Autodesk Inventor part; units mm, degrees
ref_plane "YZ Plane" through (0, 0, 0) normal (1, 0, 0) x (0, 1, 0)
ref_plane "XZ Plane" through (0, 0, 0) normal (0, 1, 0) x (-1, 0, 0)
ref_plane "XY Plane" through (0, 0, 0) normal (0, 0, 1) x (1, 0, 0)
sketch "Sketch1" plane through (0, 0, 0) normal (0, 1, 0) x (-1, 0, 0)
  line L0 (-152.4, -228.6) -> (152.4, -228.6)
  line L1 (152.4, -228.6) -> (152.4, 228.6)
  line L2 (152.4, 228.6) -> (-152.4, 228.6)
  line L3 (-152.4, 228.6) -> (-152.4, -228.6)
  line L4 (-152.4, -228.6) -> (152.4, 228.6) construction
  line L5 (152.4, -228.6) -> (-152.4, 228.6) construction
  point P0 (0, 0)
  dimension "d0" = 457.2
  dimension "d1" = 304.8
extrude "Extrusion1" add sketch "Sketch1" against normal blind 19.05
sketch "Sketch3" plane through (0, -19.05, 0) normal (0, -1, 0) x (1, 0, 0)
  line L0 (152.4, -228.6) -> (152.4, 228.6)
  line L1 (-152.4, 228.6) -> (-152.4, -228.6)
  line L2 (152.4, 228.6) -> (-152.4, 228.6)
  line L3 (-152.4, 228.6) -> (-152.4, 190.5)
  line L4 (-152.4, 190.5) -> (152.4, 190.5)
  line L5 (152.4, 190.5) -> (152.4, 228.6)
  line L6 (-152.4, -228.6) -> (152.4, -228.6)
  line L7 (152.4, -190.5) -> (-152.4, -190.5)
  line L8 (-152.4, -190.5) -> (-152.4, -228.6)
  line L9 (-152.4, -228.6) -> (152.4, -228.6)
  line L10 (152.4, -228.6) -> (152.4, -190.5)
  point P0 (0, 0)
  dimension "d4" = 38.1
  dimension "d5" = 38.1
extrude "Extrusion2" add sketch "Sketch3" along normal blind 38.1 contours L6 L1 L7 L0 | L4 L1 L2 L0
sketch "Sketch4" plane through (0, 0, 0) normal (0, 1, 0) x (1, 0, 0)
  line L0 (-152.4, -228.6) -> (152.4, -228.6)
  line L1 (-72.2315, -228.6) -> (72.2315, -228.6)
  line L2 (72.2315, -228.6) -> (72.2315, 76.2)
  line L3 (72.2315, 76.2) -> (-72.2315, 76.2)
  line L4 (-72.2315, 76.2) -> (-72.2315, -228.6)
  line L5 (-152.4, 228.6) -> (-152.4, -228.6)
  point P0 (0, 0)
  dimension "d8" = 144.463
  dimension "d9" = 304.8
  dimension "d10" = 80.1685
extrude "Extrusion3" cut sketch "Sketch4" against normal blind 19.05
sketch "Sketch5" plane through (0, 0, 0) normal (0, 1, 0) x (1, 0, 0)
  line L0 (-102.4, 228.6) -> (-65.887, 228.6)
  line L1 (-65.887, 228.6) -> (-65.887, 206.6)
  line L2 (-65.887, 206.6) -> (-102.4, 206.6)
  line L3 (-102.4, 206.6) -> (-102.4, 228.6)
  line L4 (152.4, 228.6) -> (-152.4, 228.6)
  line L5 (65.887, 228.6) -> (102.4, 228.6)
  line L6 (102.4, 228.6) -> (102.4, 206.6)
  line L7 (102.4, 206.6) -> (65.887, 206.6)
  line L8 (65.887, 206.6) -> (65.887, 228.6)
  line L9 (-152.4, 228.6) -> (-152.4, -228.6)
  line L10 (152.4, -228.6) -> (152.4, 228.6)
  point P0 (0, 0)
  point P1 (-65.887, 217.6)
  point P2 (84.1435, 228.6)
  dimension "d13" = 0
  dimension "d14" = 36.513
  dimension "d15" = 22
  dimension "d16" = 36.513
  dimension "d17" = 22
  dimension "d18" = 50
  dimension "d19" = 50
extrude "Extrusion4" cut sketch "Sketch5" against normal blind 5
properties material "Wood (Maple)"
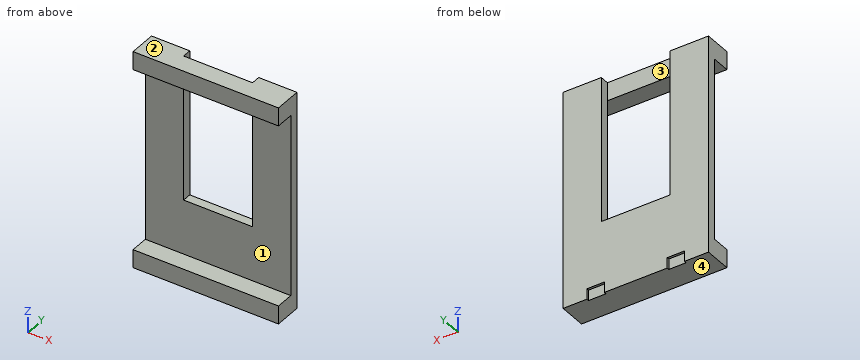
For this review, take the finished solid that the model builds, in its own axes (mm). Face numbers are marked on the shaded views. Coordinates: 2 decimals unless noted, no trailing zeros. Loops run counter-clockwise (first coordinate to the right, second up) from the corner with the lowest first, then second, coordinate; pieces in that order, holes last. Notation, with made-up numbers: (38.25, 26) - (43.25, 26) arc R28 cw to (43.25, 46) - close; hole circle Ø11 at (57.25, 51.25). An arc over 180 degrees is marked (long way). Use a Markdown table: item, result. Add a question column.
Item 1: Insertion check: pin 1 Ø9.5 at (x, y) = (-31.5, -8) entering from +Z; pin 2 Ø4 at (x, z) = (79, -97.5) entering from -Y; pin 3 Ø4 at (x, y) = (88, -1.5) entering from -Z. Each pin has a flat end and moves straight along its axis. Give the tip position at first contact, or say it passes through.
Item 2: Mouldability with a two-part tool opening along Z and no side actions: class the marked faces 1, 2, 3 and 4 as pulls with the +Z half, pulls with the -Z half, needs draft (parallel to the pull), parting line crosses it, or undercut.
Item 3: For line 1 (Z direction, x = 124, y = -51.5); line 2 (Y direction, x = -100, z = -97.5); line 3 (X direction, y = -6, z = -23), list the stretches that pass through material, from the lowest coordinate up.
Item 4: We need section A-A (y = -32.5). Give the boundary of the cut face in (x, z).
Item 5: We need section B-B (x = 2). Give the boundary of the cut face in (y, z).
Item 6: We need section D-D (x = 88.5). Give the boundary of the cut face in (y, z), and give its area (3 significant figures).
Item 7: We need section C-C (z = 102). Give the boundary of the cut face in (x, y).
Results list:
| question | item | result |
|---|---|---|
| 1 | pin 1 | stops at z = -76.2 |
| 1 | pin 2 | stops at y = -19.05 |
| 1 | pin 3 | stops at z = -206.6 |
| 2 | face 1 | undercut |
| 2 | face 2 | pulls with the +Z half |
| 2 | face 3 | needs draft |
| 2 | face 4 | pulls with the -Z half |
| 3 | line 1 | z = -228.6 to -190.5, 190.5 to 228.6 |
| 3 | line 2 | y = -19.05 to 0 |
| 3 | line 3 | x = -152.4 to -72.23, 72.23 to 152.4 |
| 4 | outline | (-152.4, -228.6) - (152.4, -228.6) - (152.4, -190.5) - (-152.4, -190.5) - close; (-152.4, 190.5) - (152.4, 190.5) - (152.4, 228.6) - (-152.4, 228.6) - close |
| 5 | outline | (-57.15, -228.6) - (0, -228.6) - (0, -76.2) - (-19.05, -76.2) - (-19.05, -190.5) - (-57.15, -190.5) - close; (-57.15, 190.5) - (-19.05, 190.5) - (-19.05, 228.6) - (-57.15, 228.6) - close |
| 6 | outline | (-57.15, -228.6) - (-5, -228.6) - (-5, -206.6) - (0, -206.6) - (0, 228.6) - (-57.15, 228.6) - (-57.15, 190.5) - (-19.05, 190.5) - (-19.05, -190.5) - (-57.15, -190.5) - close |
| 6 | area | 11,500 mm^2 |
| 7 | outline | (-152.4, -19.05) - (-72.23, -19.05) - (-72.23, 0) - (-152.4, 0) - close; (72.23, -19.05) - (152.4, -19.05) - (152.4, 0) - (72.23, 0) - close |
